Work out the finished part from the listing and answer in its coordinate system (mm). A direction names the side the tool comes from. Round coordinates to 2 decimals unless told otherwise and drop trailing zeros. Write each loop counter-clockwise with the first axis right and the second up, starting at its lowest first coordinate (ties: lowest second). Pieces come first, ordered by that corner, then holes. Notation, with made-up numbers: M -15.75,54.25 L 27.25,54.25 A18 ccw 27.25,73.25 Z; hole C 65.5,79 d10. An arc over 180 degrees is marked long. One line per item, written item: value. Start each with the question number.
Q1. Find section D-D (y = -42). Write down the section's boundary in (x, z).
Q2. The mould has two halves that part along X. Classify faces 3 (the cylindrical face through (-16.164, 22.772, 0.035)), 4 (the flat face through (35, -1, 0)), 5 (the flat face through (0, 1, 2.5)): released by +X, released by -X, zero draft, split by the parting line, or undercut.
Q3. Find section A-A (y = 47.5). Write down the section's boundary in (x, z), and give its area (3 significant figures).
Q4. Find section C-C (x = -31.25). Write down the section's boundary in (y, z).
Q5. Given pin 1 Ø1.8 at (x, y) = (-23, -18) entering from -Z; pin 2 Ø3.5 at (x, y) = (23, -18) entering from -Z, each flat-ended and moving along its own axis, determine where each tip first touches the part or whether it passes through.
Q6. Find section B-B (x = 7.5). Write down the section's boundary in (y, z), and give its area (3 significant figures).
Q7. A tool of negligible diameter and unlimited length cuts with its end or side. For faces 1 (the flat face through (0, 1, -2.5)), 2 (the flat face through (-21, -42, 0)), from which of +Z, -Z, +X, -X, +Y, -Y can it reach the whole face along a straight path? Write none if from no direction.
Q8. Consider probe 1 along X at (y, z) = (-47.5, 0.25); probe 2 along Y at (x, z) = (-23, 0.05); probe 3 along Y at (x, z) = (-12.5, 0.85). Determine where each line is inside the solid, lowest interval first.
from build123d import *

# Parameters (mm, degrees)
SKETCH1_W           = 70
SKETCH1_H           = 100
BOSS_EXTRUDE1_DEPTH = 2.5
SKETCH2_R           = 1.5
CUT_EXTRUDE1_DEPTH  = 11
SKETCH3_R           = 1.5
SKETCH3_W           = 40
SKETCH3_H           = 4
CUT_EXTRUDE2_DEPTH  = 10


with BuildPart() as part:
    # Sketch1 → Boss-Extrude1 (new, symmetric)
    with BuildSketch(Plane.XY):
        Rectangle(SKETCH1_W, SKETCH1_H)
    extrude(amount=BOSS_EXTRUDE1_DEPTH, both=True)

    # Sketch2 → Cut-Extrude1 (cut)
    with BuildSketch(Plane.XY.offset(2.5)):
        with Locations((0, 47.5)):
            Circle(SKETCH2_R)
        with Locations((-31.25, 47.5)):
            Circle(SKETCH2_R)
        with Locations(Location((31.25, 47.5, 0), (0, 0, 180))):
            Circle(SKETCH2_R)
    cut_extrude1 = extrude(amount=-CUT_EXTRUDE1_DEPTH, mode=Mode.SUBTRACT)

    # Mirror1: Cut-Extrude1 across plane
    add(cut_extrude1.mirror(Plane.ZX), mode=Mode.SUBTRACT)

    # Sketch3 → Cut-Extrude2 (cut)
    with BuildSketch(Plane.XY.offset(2.5)):
        with Locations((-17.594978519, 15.321286244)):
            Circle(SKETCH3_R)
        with Locations((-17.594978519, 22.321286244)):
            Circle(SKETCH3_R)
        with Locations((-17.594978519, 8.321286244)):
            Circle(SKETCH3_R)
        with Locations(Location((17.594978519, 8.321286244, 0), (0, 0, 180))):
            Circle(SKETCH3_R)
        with Locations(Location((17.594978519, 15.321286244, 0), (0, 0, 180))):
            Circle(SKETCH3_R)
        with Locations(Location((17.594978519, 22.321286244, 0), (0, 0, 180))):
            Circle(SKETCH3_R)
        with Locations((-23, -18)):
            Circle(SKETCH3_R)
        with Locations(Location((23, -18, 0), (0, 0, 180))):
            Circle(SKETCH3_R)
        with Locations((23, -42)):
            Circle(SKETCH3_R)
        with Locations(Location((-23, -42, 0), (0, 0, 180))):
            Circle(SKETCH3_R)
        with Locations((-1, -42)):
            Rectangle(SKETCH3_W, SKETCH3_H)
        with Locations((-1, -18)):
            Rectangle(SKETCH3_W, SKETCH3_H)
    extrude(amount=-CUT_EXTRUDE2_DEPTH, mode=Mode.SUBTRACT)


solid = part.part
The answers:
1. outline: M -35,-2.5 L -24.5,-2.5 L -24.5,2.5 L -35,2.5 Z; M -21.5,-2.5 L -21,-2.5 L -21,2.5 L -21.5,2.5 Z; M 19,-2.5 L 21.5,-2.5 L 21.5,2.5 L 19,2.5 Z; M 24.5,-2.5 L 35,-2.5 L 35,2.5 L 24.5,2.5 Z
2. face 3: undercut
2. face 4: released by +X
2. face 5: zero draft
3. outline: M -35,-2.5 L -32.75,-2.5 L -32.75,2.5 L -35,2.5 Z; M -29.75,-2.5 L -1.5,-2.5 L -1.5,2.5 L -29.75,2.5 Z; M 1.5,-2.5 L 29.75,-2.5 L 29.75,2.5 L 1.5,2.5 Z; M 32.75,-2.5 L 35,-2.5 L 35,2.5 L 32.75,2.5 Z
3. area: 305 mm2
4. outline: M -50,-2.5 L -49,-2.5 L -49,2.5 L -50,2.5 Z; M -46,-2.5 L 46,-2.5 L 46,2.5 L -46,2.5 Z; M 49,-2.5 L 50,-2.5 L 50,2.5 L 49,2.5 Z
5. pin 1: through
5. pin 2: z = -2.5
6. outline: M -50,-2.5 L -44,-2.5 L -44,2.5 L -50,2.5 Z; M -40,-2.5 L -20,-2.5 L -20,2.5 L -40,2.5 Z; M -16,-2.5 L 50,-2.5 L 50,2.5 L -16,2.5 Z
6. area: 460 mm2
7. face 1: -Z, +X, -X, +Y, -Y
7. face 2: +Z, -Z
8. probe 1: -35 to -32.75, -29.75 to -1.5, 1.5 to 29.75, 32.75 to 35
8. probe 2: -50 to -43.5, -40.5 to -19.5, -16.5 to 50
8. probe 3: -50 to -44, -40 to -20, -16 to 50
